Answer from the drawing. Dimensions are ordinates in mm from the lowest x, y and z of the part. A direction names the side the tool comes from. Coordinates: 2 decimals unless noted, no trailing zeros. Loops run counter-clockwise (first coordinate to the right, second up) from the corner with the lowest first, then second, coordinate; pieces in that order, holes last. Notation, with made-up numbers: (-37.75, 87) -> (-21.75, 87) arc R30 cw to (-21.75, 109) -> close; hole circle Ø6 at (-21.75, -22.75). An arc over 180 degrees is marked (long way). Use a Markdown table: item, result.
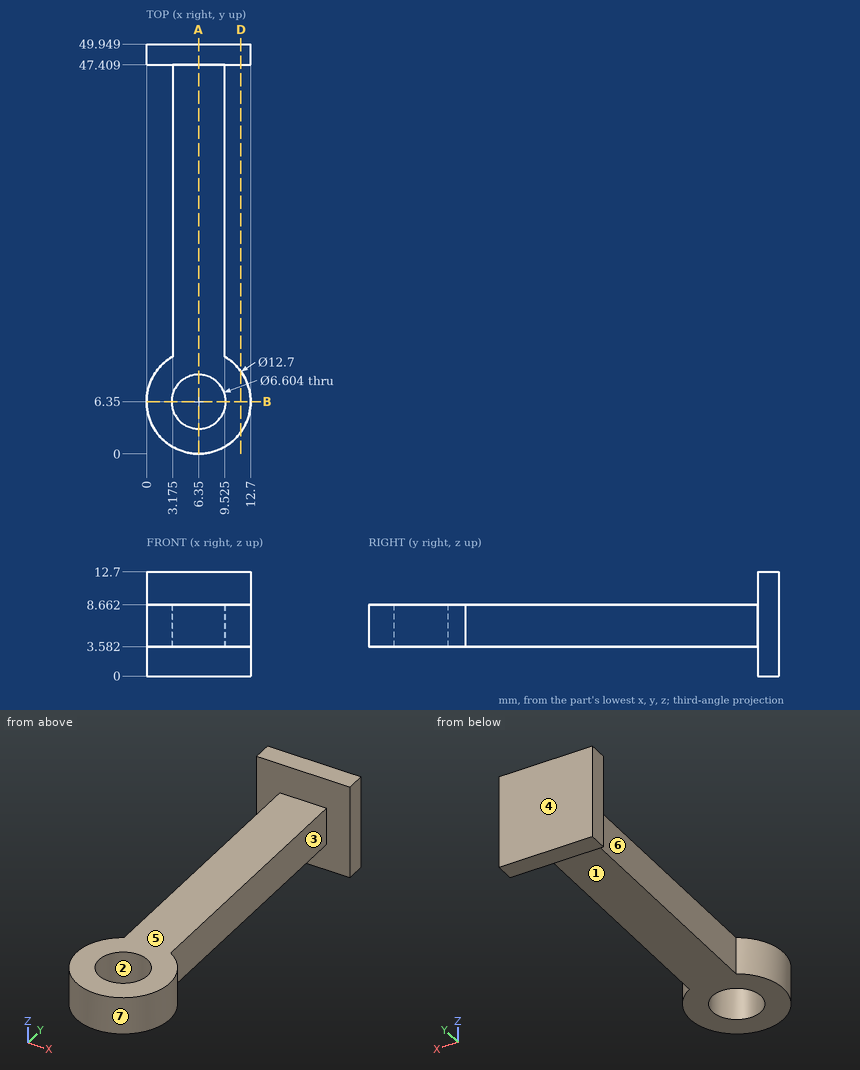
Q1. Section D-D on x = 11.5 is taken. Determine the outline of the cut face in (y, z) (1 decimal).
Solved:
| item | result |
|---|---|
| outline | (2.6, 3.6) -> (10.1, 3.6) -> (10.1, 8.7) -> (2.6, 8.7) -> close; (47.4, 0) -> (49.9, 0) -> (49.9, 12.7) -> (47.4, 12.7) -> close |
Q2. Given pin 1 Ø3 at (x, z) = (9, 4) entering from -Y (3 decimals); pin 2 Ø7.5 at (x, y) = (6.35, 6.35) entering from -Z; pin 3 Ø4 at (y, z) = (31.5, 5) entering from -X (3 decimals), each flat-ended and moving along its own axis, determine where each tip first touches the part or whether it passes through.
Solved:
| item | result |
|---|---|
| pin 1 | y = 0.105 |
| pin 2 | z = 3.58 |
| pin 3 | x = 3.175 |
Q3. Consider line 1 (Y direction, x = 6.35, z = 4.9); line 2 (Y direction, x = 9.5, z = 10.5); line 3 (Z direction, x = 8, y = 32.5). Determine where each line is inside the solid, lowest interval first. Write a range as [from, to].
Solved:
| item | result |
|---|---|
| line 1 | [0, 3.05], [9.65, 49.95] |
| line 2 | [47.41, 49.95] |
| line 3 | [3.58, 8.66] |
Q4. Section B-B on y = 6.35 is taken. Determine the outline of the cut face in (x, z), and give its area (3 significant figures).
Solved:
| item | result |
|---|---|
| outline | (0, 3.58) -> (3.05, 3.58) -> (3.05, 8.66) -> (0, 8.66) -> close; (9.65, 3.58) -> (12.7, 3.58) -> (12.7, 8.66) -> (9.65, 8.66) -> close |
| area | 31.0 mm² |
Q5. Section A-A on x = 6.35 is taken. Determine the outline of the cut face in (y, z).
Solved:
| item | result |
|---|---|
| outline | (0, 3.58) -> (3.05, 3.58) -> (3.05, 8.66) -> (0, 8.66) -> close; (9.65, 3.58) -> (47.41, 3.58) -> (47.41, 0) -> (49.95, 0) -> (49.95, 12.7) -> (47.41, 12.7) -> (47.41, 8.66) -> (9.65, 8.66) -> close |
Q6. Determine the mould class of the marked faces 4, 5, 6 and 7 for opening direction Y: pulls with the +Y half, pulls with the -Y half, needs draft (parallel to the pull), parting line crosses it, or undercut.
Solved:
| item | result |
|---|---|
| face 4 | pulls with the +Y half |
| face 5 | needs draft |
| face 6 | undercut |
| face 7 | undercut |
Q7. For the marked faces 1, 2 and 3, determine the directions among +Z, -Z, +X, -X, +Y, -Y from which every point of the face is accessible in a straight line to the end or side of a thin tool.
Solved:
| item | result |
|---|---|
| face 1 | -Z, +X, -X, -Y |
| face 2 | +Z, -Z |
| face 3 | +Z, -Z, +X |
